Job drawing, mm, ordinate dimensions from the low corner. One solid piece. A direction names the side the tool comes from. Round coordinates to 2 decimals unless told otherwise and drop trailing zeros. Write each loop counter-clockwise with the first axis right and the second up, starting at its lowest first coordinate (ties: lowest second). Pieces come first, ordered by that corner, then holes.
1) Saw through at B-B on x = 6.5. Write the cut outline in (y, z) (1 decimal).
2) Flat gauge pins, fed straight in: pin 1 (1.5 mm diameter, centred on y = 4, z = 0.5, fed in from +X) (1 decimal); pin 2 (2 mm diameter, centred on x = 6.42, y = 7.75, fed in from +Z); pin 3 (1.9 mm diameter, centred on x = 5.5, y = 7.5, fed in from +Z). Where does each tip first touch, or does it go through?
3) Drill centre lines: L1, parallel to Z at x = 9, y = 6.75; L2, parallel to X at y = 17.5, z = 3.95 (1 decimal); L3, parallel to Y at x = 8.5, z = 2.8. Where is each one in solid material? Low to high.
4) Which spindle directions (+Z, -Z, +X, -X, +Y, -Y) get a long thin tool onto all of the face, cutting with end or side? Do the marked faces 1 and 2. Say none if no direction does.
5) Saw through at A-A on y = 16.75. Write the cut outline in (x, z), and give its area (3 significant figures).
6) Pull direction X, two halves, no side cores. Call the marked faces 3, 4, 5 and 6: +X half, -X half, draft (parallel to the pull), parting line (faces both ways), or undercut.
7) Saw through at D-D on y = 5.5. Write the cut outline in (x, z), and give its area (3 significant figures).
8) Saw through at C-C on z = 4.1. Count the separate pieces of the cut face and the enclosed holes in it, and give its area (3 significant figures).
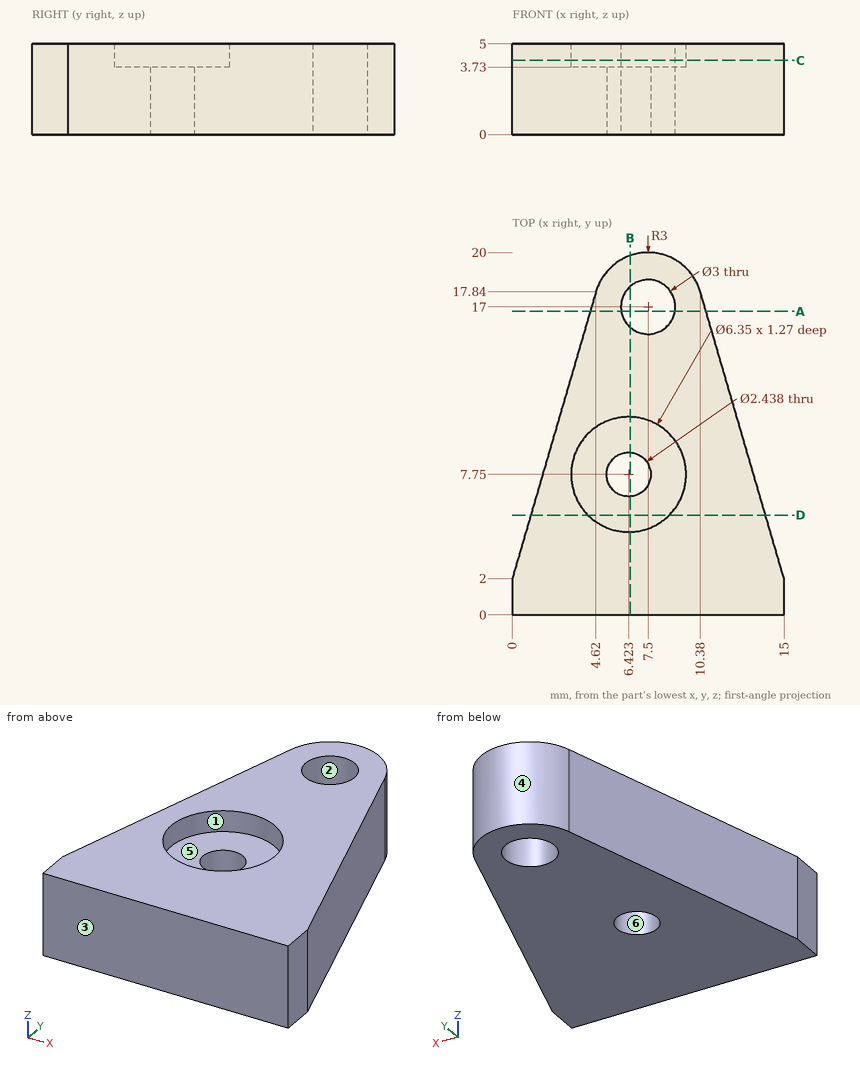
Completed:
1. outline: (0, 0) - (6.5, 0) - (6.5, 3.7) - (4.6, 3.7) - (4.6, 5) - (0, 5) - close; (9, 0) - (15.9, 0) - (15.9, 5) - (10.9, 5) - (10.9, 3.7) - (9, 3.7) - close; (18.1, 0) - (19.8, 0) - (19.8, 5) - (18.1, 5) - close
2. pin 1: stops at x = 14.6
2. pin 2: passes through
2. pin 3: stops at z = 3.73
3. L1: z = 0 to 3.73
3. L2: x = 4.5 to 6.1, 8.9 to 10.5
3. L3: y = 0 to 15.88, 18.12 to 19.83
4. face 1: +Z
4. face 2: +Z, -Z
5. outline: (4.3, 0) - (6.02, 0) - (6.02, 5) - (4.3, 5) - close; (8.98, 0) - (10.7, 0) - (10.7, 5) - (8.98, 5) - close
5. area: 17.2 mm2
6. face 3: draft
6. face 4: parting line
6. face 5: undercut
6. face 6: undercut
7. outline: (1.02, 0) - (13.98, 0) - (13.98, 5) - (8.66, 5) - (8.66, 3.73) - (4.18, 3.73) - (4.18, 5) - (1.02, 5) - close
7. area: 59.1 mm2
8. separate pieces: 1
8. enclosed holes: 2
8. area: 165 mm2
